Source: CAD feature listing. Evaluate the final solid. Frame: model axes, mm. Coordinates: 2 decimals unless noted, no trailing zeros. Loops run counter-clockwise (first coordinate to the right, second up) from the corner with the lowest first, then second, coordinate; pieces in that order, holes last. Notation, with made-up numbers: M 52,-18 L 81,-18 A20 cw 81,15 Z; hole C 78.25,2.25 d7. An arc over 180 degrees is marked long. Write each question's results on one line, items separated by ' | '. Start each with the question number.
Autodesk Inventor part; units mm, degrees
ref_plane "YZ Plane" through (0, 0, 0) normal (1, 0, 0) x (0, 1, 0)
ref_plane "XZ Plane" through (0, 0, 0) normal (0, 1, 0) x (-1, 0, 0)
ref_plane "XY Plane" through (0, 0, 0) normal (0, 0, 1) x (1, 0, 0)
sketch "Sketch1" plane through (0, 0, 0) normal (0, 0, 1) x (1, 0, 0)
  line L0 (-24, 48) -> (-24, 51)
  line L1 (-24, 51) -> (-40, 51)
  line L2 (-40, 51) -> (-40, 48)
  line L3 (0, 32) -> (3, 32)
  line L4 (3, 32) -> (3, 16)
  line L5 (3, 16) -> (0, 16)
  line L6 (-40, 0) -> (-40, -3)
  line L7 (-40, -3) -> (-24, -3)
  line L8 (-24, -3) -> (-24, 0)
  line L9 (-64, 16) -> (-67, 16)
  line L10 (-67, 16) -> (-67, 32)
  line L11 (-67, 32) -> (-64, 32)
  line L12 (-64, 48) -> (-40, 48)
  line L13 (-24, 48) -> (0, 48)
  line L14 (-64, 0) -> (-64, 16)
  line L15 (-64, 32) -> (-64, 48)
  line L16 (0, 0) -> (-24, 0)
  line L17 (-40, 0) -> (-64, 0)
  line L18 (0, 48) -> (0, 32)
  line L19 (0, 16) -> (0, 0)
  point P0 (0, 0)
  dimension "d3" = 16
  dimension "d4" = 16
  dimension "d8" = 64
  dimension "d9" = 48
  dimension "d10" = 3
  dimension "d11" = 3
  dimension "d12" = 24
  dimension "d13" = 24
  dimension "d14" = 16
  dimension "d15" = 3
extrude "Plate1" add sketch "Sketch1" along normal blind 3
equation "\"d16\" = Thickness"
equation "\"BendRadius\" = Thickness"
equation "\"BendReliefWidth\" = Thickness"
equation "\"BendReliefDepth\" = 0.5 * Thickness"
equation "\"CornerReliefSize\" = 4 * Thickness"
equation "\"MinimumRemnant\" = 2 * Thickness"
equation "\"TransitionRadius\" = BendRadius"
equation "\"JacobiRadiusSize\" = BendRadius"
equation "\"GapSize\" = Thickness"
properties part number "front plate" material "Hardboard"
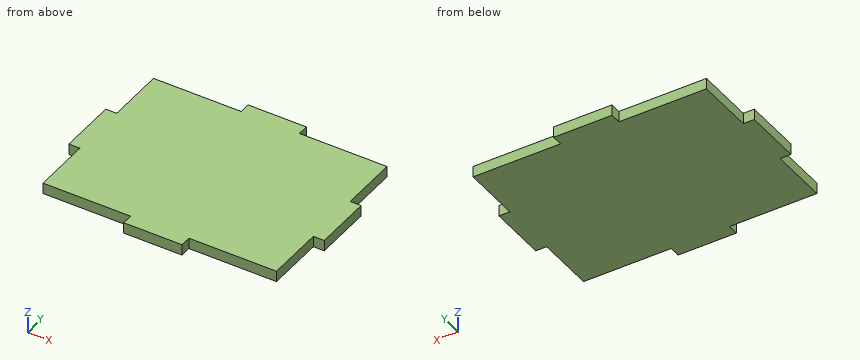
Item 1: Cut plane B-B (y = 40). Output: boundary loops of the cut face in (x, z).
Item 2: Cut plane C-C (x = -48.5). Output: boundary loops of the cut face in (y, z).
Item 3: First-contact query: pin 1 Ø6 at (x, y) = (-37, 32.5) entering from -Z; pin 2 Ø1.5 at (y, z) = (11, 2) entering from +X; pin 3 Ø0.9 at (x, z) = (-16.5, 1) entering from -Y; pin 4 Ø0.9 at (x, z) = (-65, 1) entering from -Y. Flat tips, straight axial feed; report the tip coordinate or a pass-through.
Item 4: Line query: probe 1 along X at (y, z) = (-1, 0.6); probe 2 along Y at (x, z) = (-6, 1.25); probe 3 along X at (y, z) = (33.5, 2.5). Output: solid intervals per line, ascending.
Item 5: Cut plane A-A (z = 1.6). Output: boundary loops of the cut face in (x, y), then the cut area to 3 significant figures.
Response values:
1) outline: M -64,0 L 0,0 L 0,3 L -64,3 Z
2) outline: M 0,0 L 48,0 L 48,3 L 0,3 Z
3) pin 1: stops at z = 0 | pin 2: stops at x = 0 | pin 3: stops at y = 0 | pin 4: stops at y = 16
4) probe 1: x = -40 to -24 | probe 2: y = 0 to 48 | probe 3: x = -64 to 0
5) outline: M -67,16 L -64,16 L -64,0 L -40,0 L -40,-3 L -24,-3 L -24,0 L 0,0 L 0,16 L 3,16 L 3,32 L 0,32 L 0,48 L -24,48 L -24,51 L -40,51 L -40,48 L -64,48 L -64,32 L -67,32 Z | area: 3,260 mm2
